The listing builds one solid part. Answer for the finished solid, in the listing's coordinates (mm). A direction names the side the tool comes from. Coordinates: 2 decimals unless noted, no trailing zeros. Loops run counter-clockwise (first coordinate to the right, second up) from the corner with the lowest first, then second, coordinate; pieces in that order, holes last. Notation, with made-up numbers: (45, 64) - (75, 64) arc R14 cw to (75, 78) - close; hole circle Ø7 at (-10.5, 68). An arc over 180 degrees is marked (long way). Use one line per item in the form item = value. Start each with the question number.
```python
from build123d import *

# Parameters (mm, degrees)
F0_W          = 100
F0_H          = 200
F1_DEPTH      = 4
F2_W          = 78
F2_H          = 55.5
F2_R          = 2
F3_DEPTH      = 25
F5_DEPTH      = 200
F6_W          = 100
F6_H          = 8
F7_DEPTH      = 4
F8_R          = 2
F9_DEPTH      = 200
F9_DEPTH_BACK = 200


with BuildPart() as f1:
    # F0 (on Top) → F1 (new body)
    with BuildSketch(Plane.XY):
        with Locations((4.999995, 100)):
            Rectangle(F0_W, F0_H)
    extrude(amount=F1_DEPTH)

    # F2 (on face) → F3 (cut)
    with BuildSketch(Plane.XY.offset(4)):
        with Locations((5.131312, 127.75)):
            Rectangle(F2_W, F2_H)
        with Locations((-37.500005, 98.25)):
            Circle(F2_R)
        with Locations((-37.500005, 157.25)):
            Circle(F2_R)
        with Locations((47.499995, 157.25)):
            Circle(F2_R)
        with Locations((47.499995, 98.25)):
            Circle(F2_R)
    extrude(amount=-F3_DEPTH, mode=Mode.SUBTRACT)

    # F4 (on face) → F5 (join)
    with BuildSketch(Plane.XZ):
        Polygon((-45.000005, 3), (-45.000005, 4), (-65.000005, 3), align=None)
        Polygon((74.999995, 3), (54.999995, 4), (54.999995, 3), align=None)
    extrude(amount=-F5_DEPTH)

    # F6 (on face) → F7 (join)
    with BuildSketch(Plane(origin=(0, 0, 0), x_dir=(1, 0, 0), z_dir=(0, 0, -1))):
        with Locations((4.999995, -169)):
            Rectangle(F6_W, F6_H)
    extrude(amount=F7_DEPTH)

    # F8 (on face) → F9 (cut, two sides)
    with BuildSketch(Plane.YZ.offset(54.999995)) as f9_sk:
        with Locations((169, 2.8)):
            Circle(F8_R)
    extrude(amount=F9_DEPTH, mode=Mode.SUBTRACT)
    extrude(f9_sk.sketch, amount=-F9_DEPTH_BACK, mode=Mode.SUBTRACT)


solid = f1.part
```
(1) Determine the mould class of faces 1 (the face through (4, 165, -2)), 2 (the face through (4, 186, 4)), 3 (the face through (5, 155.5, 2)), 4 (the face through (4, 173, -2)) for opening direction Y: +Y half, -Y half, draft (parallel to the pull), parting line (faces both ways), or undercut.
(2) Each of these flat-tipped pins is pushed along its axis until it touches: pin 1 Ø1.2 at (y, z) = (117, 2) entering from +X; pin 2 Ø2.5 at (x, y) = (47.5, 98.25) entering from +Z; pin 3 Ø2 at (x, y) = (5.5, 27.5) entering from -Z; pin 4 Ø22 at (x, y) = (64, 178.5) entering from -Z. Where does it stop, or does it pass through?
(3) A cutting plane is placed at A-A (y = 127.5). Determine the outline of the cut face in (x, z).
(4) A cutting plane is placed at D-D (z = -2.25). Determine the outline of the cut face in (x, y).
(5) A cutting plane is placed at B-B (x = 39.5). Determine the outline of the cut face in (y, z), then the cut area to 3 significant figures.
(6) For faces 5 (the face through (65, 82, 3)), 6 (the face through (-33.869, 127, 2)), 7 (the face through (4, 65, 0)), 8 (the face through (4, 187, 0)), 9 (the face through (-55, 185, 3)), determine the directions among +Z, -Z, +X, -X, +Y, -Y from which every point of the face is accessible in a straight line to the end or side of a thin tool.
(7) A cutting plane is placed at C-C (y = 179). Determine the outline of the cut face in (x, z).
(8) Find the intervals of material crossed by probe 1 along Y at (x, z) = (32, 2.8); probe 2 along X at (y, z) = (157.25, 0.95); probe 3 along Y at (x, z) = (42, 2), in increasing order. Write a range as from..to.
Evaluation:
q1.face_1 = -Y half
q1.face_2 = draft
q1.face_3 = undercut
q1.face_4 = +Y half
q2.pin_1 = 55
q2.pin_2 = through
q2.pin_3 = 0
q2.pin_4 = -4
q3.outline = (-65, 3) - (-45, 3) - (-45, 0) - (-33.87, 0) - (-33.87, 4) - (-45, 4) - close; (44.13, 0) - (55, 0) - (55, 3) - (75, 3) - (55, 4) - (44.13, 4) - close
q4.outline = (-45, 165) - (55, 165) - (55, 173) - (-45, 173) - close
q5.outline = (0, 0) - (100, 0) - (100, 4) - (0, 4) - close; (155.5, 0) - (165, 0) - (165, -4) - (173, -4) - (173, 0) - (200, 0) - (200, 4) - (170.6, 4) arc R2 cw (long way) to (167.4, 4) - (155.5, 4) - close
q5.area = 599 mm^2
q6.face_5 = -Z, +X, +Y, -Y
q6.face_6 = +Z, -Z
q6.face_7 = -Z, +X, -X, -Y
q6.face_8 = -Z, +X, -X, +Y
q6.face_9 = -Z, -X, +Y, -Y
q7.outline = (-65, 3) - (-45, 3) - (-45, 0) - (55, 0) - (55, 3) - (75, 3) - (55, 4) - (-45, 4) - close
q8.probe_1 = 0..100, 155.5..167, 171..200
q8.probe_2 = -45..-39.5, -35.5..45.5, 49.5..55
q8.probe_3 = 0..100, 155.5..167.17, 170.83..200
